Design review of the part built by this model. Coordinates are the model's own, in mm. Coordinates: 2 decimals unless noted, no trailing zeros. Write each loop counter-clockwise with the first axis right and the second up, starting at its lowest first coordinate (ties: lowest second). Pieces come first, ordered by that corner, then holes. Notation, with made-up numbers: M 3,-24 L 60,-24 A32 cw 60,15 Z; hole C 16.5,-8 d3. An arc over 180 degrees is marked long. One line per question, with ' | ' between items.
from build123d import *

# Parameters (mm, degrees)
BOSS_EXTRUDE1_DEPTH = 10
SKETCH2_R           = 5
CUT_EXTRUDE1_DEPTH  = 10
SKETCH3_R           = 12
BOSS_EXTRUDE2_DEPTH = 5


with BuildPart() as part:
    # Sketch1 → Boss-Extrude1 (new body)
    with BuildSketch(Plane.XY):
        with BuildLine():
            Line((-82.009618943, -15), (-112.009618943, -66.961524227))
            ThreePointArc((-112.009618943, -66.961524227), (-132.5, -72.451905284), (-137.990381057, -51.961524227))
            Line((-137.990381057, -51.961524227), (-107.990381057, 0))
            ThreePointArc((-107.990381057, 0), (-97.009618943, 10.980762114), (-82.009618943, 15))
            Line((-82.009618943, 15), (0, 15))
            Line((0, 15), (157.009618943, 15))
            ThreePointArc((157.009618943, 15), (172.009618943, 10.980762114), (182.990381057, 0))
            Line((182.990381057, 0), (262.990381057, -138.564064606))
            ThreePointArc((262.990381057, -138.564064606), (257.5, -159.054445662), (237.009618943, -153.564064606))
            Line((237.009618943, -153.564064606), (157.009618943, -15))
            Line((157.009618943, -15), (0, -15))
            Line((0, -15), (-82.009618943, -15))
        make_face()
    extrude(amount=BOSS_EXTRUDE1_DEPTH)

    # Sketch2 → Cut-Extrude1 (cut)
    with BuildSketch(Plane.XY.offset(10)):
        with Locations((-125, -59.461524227)):
            Circle(SKETCH2_R)
        with Locations((250, -146.064064606)):
            Circle(SKETCH2_R)
        Circle(SKETCH2_R)
    extrude(amount=-CUT_EXTRUDE1_DEPTH, mode=Mode.SUBTRACT)

    # Sketch3 → Boss-Extrude2 (add)
    with BuildSketch(Plane(origin=(0, 0, 0), x_dir=(-1, 0, 0), z_dir=(0, 0, -1))):
        Circle(SKETCH3_R)
    extrude(amount=BOSS_EXTRUDE2_DEPTH)


solid = part.part
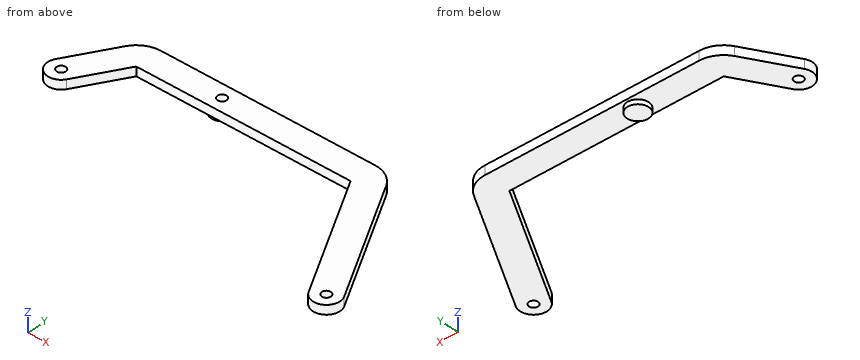
1. Take a section at B-B (x = -125). Write out the cut boundary in (y, z), then the cut area to 3 significant figures.
Answer sheet:
outline: M -74.46,0 L -64.46,0 L -64.46,10 L -74.46,10 Z; M -54.46,0 L -29.46,0 L -29.46,10 L -54.46,10 Z | area: 350 mm^2
2. Insertion check: pin 1 Ø5 at (x, y) = (-2.5, -1.5) entering from +Z; pin 2 Ø9 at (x, y) = (250, -146.06) entering from -Z; pin 3 Ø1 at (x, z) = (185.5, 7.5) entering from +Y; pin 4 Ø9 at (x, y) = (0, 0) entering from +Z. Each pin has a flat end and moves straight along its axis. Give the tip position at first contact, or say it passes through.
Answer sheet:
pin 1: z = 10 | pin 2: through | pin 3: y = -3.48 | pin 4: z = 0
3. Take a section at D-D (x = 82). Write out the cut boundary in (y, z), then the cut area to 3 significant figures.
Answer sheet:
outline: M -15,0 L 15,0 L 15,10 L -15,10 Z | area: 300 mm^2
4. Take a section at C-C (z = 2.5). Write out the cut boundary in (x, y), then the cut area to 3 significant figures.
Answer sheet:
outline: M -137.99,-51.96 A15 ccw -112.01,-66.96 L -82.01,-15 L 157.01,-15 L 237.01,-153.56 A15 ccw 262.99,-138.56 L 182.99,0 A30 ccw 157.01,15 L -82.01,15 A30 ccw -107.99,0 Z; hole C -125,-59.46 d10; hole C 0,0 d10; hole C 250,-146.06 d10 | area: 15,200 mm^2
5. Take a section at A-A (y = -70.5). Write out the cut boundary in (x, z).
Answer sheet:
outline: M -135.16,0 L -114.84,0 L -114.84,10 L -135.16,10 Z; M 189.05,0 L 223.69,0 L 223.69,10 L 189.05,10 Z
6. To check wall thickness, follow line 1 along Y through (x, z) = (0, 6.75); line 2 along Y through (x, z) = (34, 9.5); line 3 along X through (y, z) = (-143, 6.75). State the ranges of each line that lie inside material, in increasing order. Write a range as [from, to].
Answer sheet:
line 1: [-15, -5], [5, 15] | line 2: [-15, 15] | line 3: [230.91, 246.05], [253.95, 264.68]
